Here's how the part is built. I have some questions about the finished solid (model axes, mm). A direction names the side the tool comes from. Round coordinates to 2 decimals unless told otherwise and drop trailing zeros. Loops run counter-clockwise (first coordinate to the right, second up) from the corner with the lowest first, then second, coordinate; pieces in that order, holes last. Notation, with made-up numbers: M -11,20.25 L 31,20.25 A20 ccw 31,25.25 Z; hole C -40,36 d7. An arc over 180 degrees is marked long. Write each question's results on one line, items separated by ' | '. Start each with the question number.
```python
from build123d import *

# Parameters (mm, degrees)
SKETCH2_R          = 2.5
CUT_EXTRUDE1_DEPTH = 4.5
CUT_EXTRUDE2_REACH = 36.5
SKETCH3_R          = 2.5


with BuildPart() as part:
    # Sketch1 → Revolve1 (revolve)
    with BuildSketch(Plane.XY):
        Polygon((-14.700460829, 4.5), (-14.700460829, 12), (-1.700460829, 12), (-1.700460829, 22.5), (2.799539171, 22.5), (2.799539171, 4.5), align=None)
    revolve(axis=Axis((-11.612903226, 0, 0), (1, 0, 0)))

    # Sketch2 → Cut-Extrude1 (cut)
    with BuildSketch(Plane.ZY.offset(1.700460829)):
        with Locations((0, 17.25)):
            Circle(SKETCH2_R)
        with Locations((14.938938215, 8.625)):
            Circle(SKETCH2_R)
        with Locations((14.938938215, -8.625)):
            Circle(SKETCH2_R)
        with Locations((0, -17.25)):
            Circle(SKETCH2_R)
        with Locations((-14.938938215, -8.625)):
            Circle(SKETCH2_R)
        with Locations((-14.938938215, 8.625)):
            Circle(SKETCH2_R)
    extrude(amount=-CUT_EXTRUDE1_DEPTH, mode=Mode.SUBTRACT)

    # Sketch3 → Cut-Extrude2 (cut, up to next)
    with BuildSketch(Plane.XY.offset(12), mode=Mode.PRIVATE) as cut_extrude2_sk1:
        with Locations((-8.200460829, 0)):
            Circle(SKETCH3_R)
    cut_extrude2_tool1 = extrude(cut_extrude2_sk1.sketch, amount=-CUT_EXTRUDE2_REACH, mode=Mode.PRIVATE) & part.part
    add(cut_extrude2_tool1.solids().sort_by_distance((-8.200461, 0, 12))[0], mode=Mode.SUBTRACT)


solid = part.part
```
Item 1: If we mould it in two halves opening along Z, with no side actions, what happens to faces 1 (the face through (-8.109, -2.601, -11.715)), 2 (the face through (-1.7, -10, -10)), 3 (the face through (0.52, 19.36, 1.34))? For each: released by +Z, released by -Z, zero draft, split by the parting line, or undercut.
Item 2: If we section it at B-B on z = 0: Please give me the cut outline in (x, y), and give its area (3 significant figures).
Item 3: I need wall thicknesses on L1, parallel to X at y = -15.5, z = -6; L2, parallel to Z at x = -6, y = 2; L3, parallel to Y at x = -8.25, z = 4. Which ranges of each line are inside material? Lowest first, please.
Item 4: Which directions (+Z, -Z, +X, -X, +Y, -Y) give clear straight access to the entire face, cutting with the end or side of a thin tool? Please do faces 4 (the face through (-10.7, 0.1, 7.9)), 5 (the face through (0.52, 7.1, 12.96)).
Item 5: If we section it at D-D on z = -15.5: Please give me the cut outline in (x, y), and give its area (3 significant figures).
Item 6: If we section it at A-A on y = 0: Please give me the cut outline in (x, z).
Item 7: If we section it at C-C on x = -0.5: Please give me the cut outline in (y, z) (3 decimals).
Item 8: I'm going to push flat-ended pins straight in: pin 1 (2 mm diameter, centred on x = -4.5, y = -2, fed in from -Z); pin 2 (10 mm diameter, centred on x = -10.5, z = 5.5, fed in from -Y); pin 3 (6 mm diameter, centred on x = -3, y = -5.5, fed in from -Z). Where does each tip first touch, or does it pass through?
Numbers:
1) face 1: split by the parting line | face 2: zero draft | face 3: undercut
2) outline: M -14.7,-12 L -1.7,-12 L -1.7,-14.75 L 2.8,-14.75 L 2.8,-4.5 L -14.7,-4.5 Z; M -14.7,4.5 L 2.8,4.5 L 2.8,14.75 L -1.7,14.75 L -1.7,12 L -14.7,12 Z; M -1.7,-22.5 L 2.8,-22.5 L 2.8,-19.75 L -1.7,-19.75 Z; M -1.7,19.75 L 2.8,19.75 L 2.8,22.5 L -1.7,22.5 Z | area: 312 mm²
3) L1: -1.7 to 2.8 | L2: -11.83 to -4.03, 4.03 to 11.83 | L3: -11.31 to -2.5, 2.5 to 11.31
4) face 4: +Z | face 5: +X, -X
5) outline: M -1.7,-16.31 L 2.8,-16.31 L 2.8,-11.06 L -1.7,-11.06 Z; M -1.7,-6.19 L 2.8,-6.19 L 2.8,6.19 L -1.7,6.19 Z; M -1.7,11.06 L 2.8,11.06 L 2.8,16.31 L -1.7,16.31 Z | area: 103 mm²
6) outline: M -14.7,-12 L -1.7,-12 L -1.7,-22.5 L 2.8,-22.5 L 2.8,-4.5 L -14.7,-4.5 Z; M -14.7,4.5 L -10.7,4.5 L -10.7,12 L -14.7,12 Z; M -5.7,4.5 L 2.8,4.5 L 2.8,22.5 L -1.7,22.5 L -1.7,12 L -5.7,12 Z
7) outline: C 0,0 d45; hole C -17.25,0 d5; hole C -8.625,-14.939 d5; hole C -8.625,14.939 d5; hole C 0,0 d9; hole C 8.625,-14.939 d5; hole C 8.625,14.939 d5; hole C 17.25,0 d5
8) pin 1: z = -11.96 | pin 2: y = -11.99 | pin 3: z = -22.33
